Autodesk Inventor part; units mm, degrees
ref_plane "YZ Plane" through (0, 0, 0) normal (1, 0, 0) x (0, 1, 0)
ref_plane "XZ Plane" through (0, 0, 0) normal (0, 1, 0) x (-1, 0, 0)
ref_plane "XY Plane" through (0, 0, 0) normal (0, 0, 1) x (1, 0, 0)
sketch "スケッチ1" plane through (0, 0, 0) normal (0, 1, 0) x (-1, 0, 0)
  circle A0 centre (0, 0) radius 125
  dimension "d0" = 250
extrude "押し出し1" add sketch "スケッチ1" along normal blind 4
sketch "スケッチ2" plane through (0, 4, 0) normal (0, 1, 0) x (1, 0, 0)
  line L0 (75, -84.411) -> (-75, -84.411)
  line L1 (-75, -84.411) -> (-75, 95.589)
  line L2 (-75, 95.589) -> (75, 95.589)
  line L3 (75, 95.589) -> (75, -84.411)
  line L4 (75, -84.411) -> (-75, 95.589) construction
  line L5 (-75, -84.411) -> (75, 95.589) construction
  circle A0 centre (0, 0) radius 121.5
  line L6 (0, 0) -> (0, -125) construction
  circle A1 centre (0, 0) radius 125
  line L7 (0, 0) -> (108.2532, 62.5) construction
  line L8 (0, 0) -> (-108.2532, 62.5) construction
  circle A2 centre (-16.75, 82.589) radius 4.1
  point P0 (0, 5.589)
  dimension "d3" = 150
  dimension "d4" = 180
  dimension "d5" = 243
  dimension "d8" = 360
  dimension "d12" = 16.75
  dimension "d13" = 13
  dimension "d14" = 8.2
extrude "押し出し2" cut sketch "スケッチ2" against normal blind 4 contours A2
sketch "スケッチ4" plane through (0, 4, 0) normal (0, 1, 0) x (1, 0, 0)
  circle A0 centre (0, 0) radius 121.5
  line L0 (75, -84.411) -> (-75, -84.411)
  line L1 (-75, -84.411) -> (-75, 95.589)
  line L2 (-75, 95.589) -> (75, 95.589)
  line L3 (75, 95.589) -> (75, -84.411)
  line L4 (75, -84.411) -> (-75, 95.589) construction
  line L5 (-75, -84.411) -> (75, 95.589) construction
  line L6 (0, 0) -> (0, -29.9183)
  point P0 (0, 5.589)
  point P1 (69, -54.411)
  point P2 (69, 5.589)
  point P3 (69, 65.589)
  point P4 (-69, -54.411)
  point P5 (-69, 5.589)
  point P6 (-69, 65.589)
  dimension "d17" = 243
  dimension "d18" = 150
  dimension "d19" = 180
  dimension "d20" = 30
  dimension "d21" = 6
  dimension "d22" = 60
  dimension "d23" = 60
hole "穴1" at (69, 4, 54.411) at (69, 4, -5.589) at (69, 4, -65.589) at (-69, 4, -65.589) at (-69, 4, -5.589) at (-69, 4, 54.411) direction (0, -1, 0) diameter 3.2 end through all
sketch "スケッチ5" plane through (0, 4, 0) normal (0, 1, 0) x (1, 0, 0)
  point P0 (0, 0)
  point P1 (0, -116.86)
  point P2 (20, -116.86)
  point P3 (-20, -116.86)
  point P4 (111.2037, 41.1095)
  point P5 (91.2037, 75.7505)
  point P6 (101.2037, 58.43)
  point P7 (-91.2037, 75.7505)
  point P8 (-111.2037, 41.1095)
  point P9 (-101.2037, 58.43)
  dimension "d31" = 116.86
  dimension "d32" = 20
  dimension "d33" = 20
  dimension "d36" = 360
hole "穴2" at (20, 4, 116.86) at (-20, 4, 116.86) at (111.2037, 4, -41.1095) at (91.2037, 4, -75.7505) at (-91.2037, 4, -75.7505) at (-111.2037, 4, -41.1095) direction (0, -1, 0) diameter 3.2 depth 10
sketch "スケッチ6" plane through (0, 4, 0) normal (0, 1, 0) x (1, 0, 0)
  point P0 (0, 0)
  point P1 (0, 116.86)
  point P2 (-10, 116.86)
  point P3 (10, 116.86)
  point P4 (-106.2037, -49.7697)
  point P5 (-96.2037, -67.0903)
  point P6 (-101.2037, -58.43)
  point P7 (96.2037, -67.0903)
  point P8 (106.2037, -49.7697)
  point P9 (101.2037, -58.43)
  dimension "d45" = 116.86
  dimension "d46" = 10
  dimension "d47" = 10
  dimension "d50" = 360
hole "穴3" at (-10, 4, -116.86) at (10, 4, -116.86) at (-106.2037, 4, 49.7697) at (-96.2037, 4, 67.0903) at (96.2037, 4, 67.0903) at (106.2037, 4, 49.7697) direction (0, -1, 0) diameter 3.2 depth 10
sketch "スケッチ7" plane through (0, 4, 0) normal (0, 1, 0) x (1, 0, 0)
  circle A0 centre (-16.75, 82.589) radius 4.1
  line L0 (-16.75, 82.589) -> (-27.75, 63.5364) construction
  line L1 (-16.75, 82.589) -> (5.25, 82.589) construction
  line L2 (-27.75, 63.5364) -> (-49.4006, 76.0364)
  line L3 (-49.4006, 76.0364) -> (-6.0994, 51.0364) construction
  point P0 (0, 0)
  dimension "d59" = 22
  dimension "d60" = 120
  dimension "d61" = 25
  dimension "d62" = 50
hole "穴4" at (-49.4006, 4, -76.0364) at (-6.0994, 4, -51.0364) direction (0, -1, 0) diameter 3.2 depth 10
properties part number "中間台1"
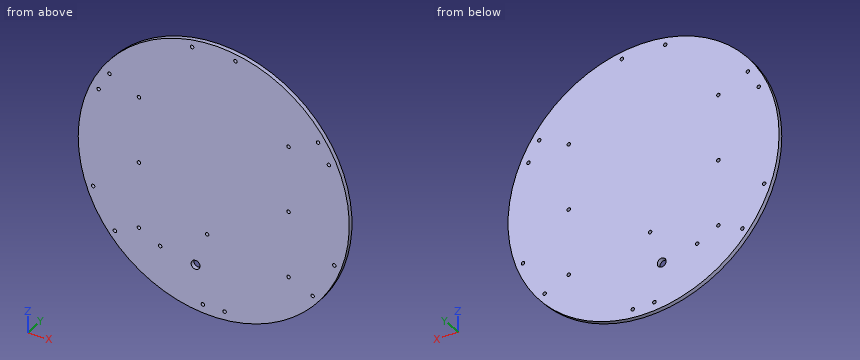
Could you check a few things on this model? Use its own coordinates, in mm. Give positions to 0.01 mm unless a question says otherwise; leave off trailing zeros. Loops run counter-clockwise (first coordinate to the right, second up) from the corner with the lowest first, then second, coordinate; pieces in that order, holes last. Notation, with made-up numbers: (67, 58.25) -> (121, 58.25) arc R7 ccw to (121, 71.25) -> close; hole circle Ø5 at (38, -20.5). An arc over 180 degrees is marked (long way). Put each result on its own line as item: value.
(1) Imagine slicing it at C-C on x = 26. Write out the boundary of the cut face in (y, z), plus the area to 3 significant figures.
Computed:
outline: (0, -122.27) -> (4, -122.27) -> (4, 122.27) -> (0, 122.27) -> close
area: 978 mm^2
(2) Imagine slicing it at B-B on z = -93.5. Write out the boundary of the cut face in (x, y), plus the area to 3 significant figures.
Computed:
outline: (-82.96, 0) -> (82.96, 0) -> (82.96, 4) -> (-82.96, 4) -> close
area: 664 mm^2
(3) I'm going to push flat-ended pins straight in: pin 1 Ø4 at (x, z) = (69, 54.411) entering from +Y; pin 2 Ø1.5 at (x, y) = (27, 3) entering from -Z. Where does each tip first touch, or does it pass through?
Computed:
pin 1: y = 4
pin 2: z = -122.21
(4) Imagine slicing it at A-A on y = 2.2. State how many separate pieces and enclosed holes the cut face has, plus the area to 3 significant figures.
Computed:
separate pieces: 1
enclosed holes: 21
area: 48,900 mm^2
(5) Please list where these lines run through material, in increasing order: probe 1 along Z at (x, y) = (-69, 1.9); probe 2 along X at (y, z) = (3.35, -6); probe 3 along X at (y, z) = (1.4, 50). Write a range as [from, to].
Computed:
probe 1: [-104.23, -67.19], [-63.99, -7.19], [-3.99, 52.81], [56.01, 104.23]
probe 2: [-124.86, -70.55], [-67.45, 67.45], [70.55, 124.86]
probe 3: [-114.56, -107.79], [-104.62, 104.62], [107.79, 114.56]
